The model under review builds one solid part; all positions refer to its coordinate system, in mm. Give positions to 0.01 mm unless a question says otherwise; leave off trailing zeros. Write each loop counter-clockwise with the first axis right and the second up, starting at its lowest first coordinate (ties: lowest second). Pieces come first, ordered by that corner, then holes. Notation, with made-up numbers: (31, 16) -> (61, 16) arc R18 ccw to (61, 36) -> close; hole circle Ø8 at (26, -11.75). An arc over 180 degrees is marked (long way). Use CSV: the item, a comma, the result in double quotes.
```python
from build123d import *

# Parameters (mm, degrees)
PAD_DEPTH       = 5
PAD001_DEPTH    = 5
SKETCH001_R     = 45
POCKET_DEPTH    = 5.001
FILLET_R        = 1
FILLET001_R     = 1
FILLET002_R     = 1
FILLET003_R     = 1
FILLET004_R     = 1
FILLET005_R     = 1
FILLET006_R     = 1
FILLET007_R     = 1
SKETCH002_R     = 2.4
POCKET001_DEPTH = 5


with BuildPart() as part:
    # Sketch → Pad (new body)
    with BuildSketch(Plane.XZ):
        with BuildLine():
            ThreePointArc((29.708208, 50.912333), (0, 55), (-29.708208, 50.912333))
            ThreePointArc((-29.708208, 50.912333), (-50.606602, 50.606602), (-50.912333, 29.708208))
            ThreePointArc((-50.912333, 29.708208), (-55, 0), (-50.912333, -29.708208))
            ThreePointArc((-50.912333, -29.708208), (-50.606602, -50.606602), (-29.708208, -50.912333))
            ThreePointArc((-29.708208, -50.912333), (0, -55), (29.708208, -50.912333))
            ThreePointArc((29.708208, -50.912333), (50.606602, -50.606602), (50.912333, -29.708208))
            ThreePointArc((50.912333, -29.708208), (55, 0), (50.912333, 29.708208))
            ThreePointArc((50.912333, 29.708208), (50.606602, 50.606602), (29.708208, 50.912333))
        make_face()
    extrude(amount=PAD_DEPTH)

    # Sketch → Pad001 (join)
    with BuildSketch(Plane.XZ):
        with BuildLine():
            ThreePointArc((29.708208, 50.912333), (0, 55), (-29.708208, 50.912333))
            ThreePointArc((-29.708208, 50.912333), (-50.606602, 50.606602), (-50.912333, 29.708208))
            ThreePointArc((-50.912333, 29.708208), (-55, 0), (-50.912333, -29.708208))
            ThreePointArc((-50.912333, -29.708208), (-50.606602, -50.606602), (-29.708208, -50.912333))
            ThreePointArc((-29.708208, -50.912333), (0, -55), (29.708208, -50.912333))
            ThreePointArc((29.708208, -50.912333), (50.606602, -50.606602), (50.912333, -29.708208))
            ThreePointArc((50.912333, -29.708208), (55, 0), (50.912333, 29.708208))
            ThreePointArc((50.912333, 29.708208), (50.606602, 50.606602), (29.708208, 50.912333))
        make_face()
    extrude(amount=PAD001_DEPTH)

    # Sketch001 (on Face5 of Pad001) → Pocket (cut, through all)
    with BuildSketch(Plane.XZ.offset(5)):
        Circle(SKETCH001_R)
    extrude(amount=-POCKET_DEPTH, mode=Mode.SUBTRACT)

    # Fillet
    fillet_edges = [part.edges().sort_by_distance(p)[0] for p in [
        (-29.708208, -2.5, 50.912333),
    ]]
    fillet(fillet_edges, radius=FILLET_R)

    # Fillet001
    fillet001_edges = [part.edges().sort_by_distance(p)[0] for p in [
        (29.708208, -2.5, 50.912333),
    ]]
    fillet(fillet001_edges, radius=FILLET001_R)

    # Fillet002
    fillet002_edges = [part.edges().sort_by_distance(p)[0] for p in [
        (50.912333, -2.5, -29.708208),
    ]]
    fillet(fillet002_edges, radius=FILLET002_R)

    # Fillet003
    fillet003_edges = [part.edges().sort_by_distance(p)[0] for p in [
        (50.912333, -2.5, 29.708208),
    ]]
    fillet(fillet003_edges, radius=FILLET003_R)

    # Fillet004
    fillet004_edges = [part.edges().sort_by_distance(p)[0] for p in [
        (29.708208, -2.5, -50.912333),
    ]]
    fillet(fillet004_edges, radius=FILLET004_R)

    # Fillet005
    fillet005_edges = [part.edges().sort_by_distance(p)[0] for p in [
        (-29.708208, -2.5, -50.912333),
    ]]
    fillet(fillet005_edges, radius=FILLET005_R)

    # Fillet006
    fillet006_edges = [part.edges().sort_by_distance(p)[0] for p in [
        (-50.912333, -2.5, 29.708208),
    ]]
    fillet(fillet006_edges, radius=FILLET006_R)

    # Fillet007
    fillet007_edges = [part.edges().sort_by_distance(p)[0] for p in [
        (-50.912333, -2.5, -29.708208),
    ]]
    fillet(fillet007_edges, radius=FILLET007_R)

    # Sketch002 (on Face19 of Fillet007) → Pocket001 (cut)
    with BuildSketch(Plane.XZ.offset(5)):
        with Locations((-42, 42)):
            Circle(SKETCH002_R)
        with Locations((42, 42)):
            Circle(SKETCH002_R)
        with Locations((42, -42)):
            Circle(SKETCH002_R)
        with Locations((-42, -42)):
            Circle(SKETCH002_R)
    extrude(amount=-POCKET001_DEPTH, mode=Mode.SUBTRACT)


solid = part.part
```
Q1. Insertion check: pin 1 (2 mm diameter, centred on x = -18, y = -1.5, fed in from +Z). The pin has a flat end and moves straight along its axis. Give the tip position at first contact, or say it passes through.
Derived:
pin 1,"stops at z = 53.68"
Q2. Consider section B-B (z = -42). Write out the cut boundary in (x, y).
Derived:
outline,"(-54.87, -5) -> (-44.4, -5) -> (-44.4, 0) -> (-54.87, 0) -> close; (-39.6, -5) -> (-16.16, -5) -> (-16.16, 0) -> (-39.6, 0) -> close; (16.16, -5) -> (39.6, -5) -> (39.6, 0) -> (16.16, 0) -> close; (44.4, -5) -> (54.87, -5) -> (54.87, 0) -> (44.4, 0) -> close"
Q3. Consider section D-D (x = -42). Write out the cut boundary in (y, z).
Derived:
outline,"(-5, -54.87) -> (0, -54.87) -> (0, -44.4) -> (-5, -44.4) -> close; (-5, -39.6) -> (0, -39.6) -> (0, -16.16) -> (-5, -16.16) -> close; (-5, 16.16) -> (0, 16.16) -> (0, 39.6) -> (-5, 39.6) -> close; (-5, 44.4) -> (0, 44.4) -> (0, 54.87) -> (-5, 54.87) -> close"
Q4. The part is to be moulded in two halves that separate along Z. For faces 1 (the cylindrical face through (0, -2, -55)), 2 (the cylindrical face through (0, -2, 55)), 3 (the flat face through (-50, 0, 1)), 4 (the cylindrical face through (41.48, -2.535, 39.657)), say which applies: pulls with the +Z half, pulls with the -Z half, needs draft (parallel to the pull), parting line crosses it, or undercut.
Derived:
face 1,"pulls with the -Z half"
face 2,"pulls with the +Z half"
face 3,"needs draft"
face 4,"undercut"
Q5. Consider section C-C (z = -8). Write out the cut boundary in (x, y).
Derived:
outline,"(-54.71, -5) -> (-44.28, -5) -> (-44.28, 0) -> (-54.71, 0) -> close; (44.28, -5) -> (54.71, -5) -> (54.71, 0) -> (44.28, 0) -> close"
Q6. To check wall thickness, follow probe 1 along Z at (x, y) = (0, -1.25); probe 2 along X at (y, z) = (-1.3, 1.5) (3 decimals); probe 3 along Z at (x, y) = (-25, -0.6). State the ranges of each line that lie inside material, in increasing order.
Derived:
probe 1,"z = -55 to -45, 45 to 55"
probe 2,"x = -54.99 to -44.975, 44.975 to 54.99"
probe 3,"z = -52.12 to -37.42, 37.42 to 52.12"
Q7. Consider section A-A (x = 0). Write out the cut boundary in (y, z).
Derived:
outline,"(-5, -55) -> (0, -55) -> (0, -45) -> (-5, -45) -> close; (-5, 45) -> (0, 45) -> (0, 55) -> (-5, 55) -> close"
